```python
from build123d import *

# Parameters (mm, degrees)
SKETCH1_R           = 4.5
BOSS_EXTRUDE1_DEPTH = 7
SKETCH2_R           = 2.5
CUT_EXTRUDE1_DEPTH  = 10.460443964
SKETCH4_W           = 3
SKETCH4_H           = 6
FILLET1_R           = 0.8


with BuildPart() as part:
    # Sketch1 → Boss-Extrude1 (new body)
    with BuildSketch(Plane(origin=(0, 0, 0), x_dir=(1, 0, 0), z_dir=(0, 1, 0))):
        with Locations(Location((0, 0, 0), (0, 0, 90))):
            Circle(SKETCH1_R)
    extrude(amount=BOSS_EXTRUDE1_DEPTH)

    # Sketch2 → Cut-Extrude1 (cut, through all)
    with BuildSketch(Plane(origin=(0, 7, 0), x_dir=(1, 0, 0), z_dir=(0, 1, 0))):
        with Locations(Location((0, 0, 0), (0, 0, 270))):
            Circle(SKETCH2_R)
    extrude(amount=-CUT_EXTRUDE1_DEPTH, mode=Mode.SUBTRACT)

    # Sweep1: sweep along a path in Sketch3
    with BuildLine(Plane(origin=(0, 3.5, 0), x_dir=(1, 0, 0), z_dir=(0, 1, 0))) as sweep1_path:
        Line((35, 6), (0, 6))
        ThreePointArc((0, 6), (-6, 0), (0, -6))
        Line((0, -6), (35, -6))
    # Sketch4 → Sweep1 (sweep)
    with BuildSketch(Plane(origin=(35, 0, 0), x_dir=(0, 0, -1), z_dir=(1, 0, 0))):
        with Locations((6, 3.5)):
            Rectangle(SKETCH4_W, SKETCH4_H)
    sweep(path=sweep1_path.line)

    # Fillet1
    fillet1_edges = [part.edges().sort_by_distance(p)[0] for p in [
        (35, 3.5, -7.5),
        (35, 6.5, -6),
        (35, 3.5, -4.5),
        (35, 0.5, -6),
        (35, 3.5, 4.5),
        (17.5, 0.5, 7.5),
        (35, 0.5, 6),
        (17.5, 6.5, 7.5),
        (35, 3.5, 7.5),
        (35, 6.5, 6),
        (-7.5, 0.5, 0),
        (-7.5, 6.5, 0),
        (17.5, 0.5, -7.5),
        (17.5, 6.5, -7.5),
    ]]
    fillet(fillet1_edges, radius=FILLET1_R)


solid = part.part
```
Here's how the part is built. I have some questions about the finished solid (model axes, mm). A direction names the side the tool comes from. Coordinates: 2 decimals unless noted, no trailing zeros. Write each loop counter-clockwise with the first axis right and the second up, starting at its lowest first coordinate (ties: lowest second). Pieces come first, ordered by that corner, then holes. Notation, with made-up numbers: (-38, 40.25) -> (18, 40.25) arc R30 cw to (18, 62.25) -> close; hole circle Ø9 at (33.25, 16.25). An arc over 180 degrees is marked (long way). Use a Markdown table: item, result. Add a question column.
(1) Please list where these lines run through material, in increasing order: line 1 (Z direction, x = 27.5, y = 4.5); line 2 (X direction, y = 5, z = 0); line 3 (Z direction, x = 3, y = 2).
(2) If we section it at C-C, the plane y = 3: Write out the boundary of the cut face in (x, z).
(3) We'd pull the mould along X, two halves only. Please class faces 1 (the cylindrical face through (-7.5, 3.53, -0.16)), 2 (the cylindrical face through (-2.44, 3.55, -0.54)), 3 (the flat face through (35, 3, 6)): +X half, -X half, draft (parallel to the pull), parting line (faces both ways), or undercut.
(4) If we section it at A-A, the plane z = 0: Write out the boundary of the cut face in (x, y).
(5) I'm going to push flat-ended pins straight in: P1, Ø3, axis at x = 0, z = 0, coming from the +Y side; P2, Ø1.5, axis at y = 3, z = -1, coming from the -X side; P3, Ø5, axis at x = 26.5, z = -4.5, coming from the +Y side; P4, Ø6, axis at x = 16, z = 2, coming from the -Y side. Where does each tip first touch, or does it pass through?
(6) For faces 4 (the cylindrical face through (34.76, 3.46, -4.73)), 5 (the cylindrical face through (34.76, 6.27, -5.58)), 6 (the flat face through (14, 6.5, -5)), which set-ups out of +Z, -Z, +X, -X, +Y, -Y let a thin tool reach every point of the face, with its end or its side?
(7) If we section it at B-B, the plane x = 27: Write out the boundary of the cut face in (y, z).
Outcome:
| question | item | result |
|---|---|---|
| 1 | line 1 | z = -7.5 to -4.5, 4.5 to 7.5 |
| 1 | line 2 | x = -7.5 to -2.5, 2.5 to 4.5 |
| 1 | line 3 | z = -7.5 to -4.5, -3.35 to 3.35, 4.5 to 7.5 |
| 2 | outline | (0, -7.5) -> (34.2, -7.5) arc R0.8 ccw to (35, -6.7) -> (35, -5.3) arc R0.8 ccw to (34.2, -4.5) -> (0, -4.5) arc R4.5 ccw to (0, 4.5) -> (34.2, 4.5) arc R0.8 ccw to (35, 5.3) -> (35, 6.7) arc R0.8 ccw to (34.2, 7.5) -> (0, 7.5) arc R7.5 ccw to start; hole circle Ø5 at (0, 0) |
| 3 | face 1 | -X half |
| 3 | face 2 | undercut |
| 3 | face 3 | +X half |
| 4 | outline | (-7.5, 1.3) arc R0.8 ccw to (-6.7, 0.5) -> (-4.5, 0.5) -> (-4.5, 0) -> (-2.5, 0) -> (-2.5, 7) -> (-4.5, 7) -> (-4.5, 6.5) -> (-6.7, 6.5) arc R0.8 ccw to (-7.5, 5.7) -> close; (2.5, 0) -> (4.5, 0) -> (4.5, 7) -> (2.5, 7) -> close |
| 5 | P1 | passes through |
| 5 | P2 | stops at x = -7.5 |
| 5 | P3 | stops at y = 6.5 |
| 5 | P4 | stops at y = 0.5 |
| 6 | face 4 | +X, +Y, -Y |
| 6 | face 5 | +Z, -Z, +X, +Y |
| 6 | face 6 | -X, +Y |
| 7 | outline | (0.5, -6.7) arc R0.8 ccw to (1.3, -7.5) -> (5.7, -7.5) arc R0.8 ccw to (6.5, -6.7) -> (6.5, -4.5) -> (0.5, -4.5) -> close; (0.5, 4.5) -> (6.5, 4.5) -> (6.5, 6.7) arc R0.8 ccw to (5.7, 7.5) -> (1.3, 7.5) arc R0.8 ccw to (0.5, 6.7) -> close |
